For this review, take the finished solid that the model builds, in its own axes (mm). A direction names the side the tool comes from. Round coordinates to 2 decimals unless told otherwise and drop trailing zeros. Order: outer loops, then holes, each group sorted by start corner. A loop starts at its lowest first (then second) coordinate and runs counter-clockwise, first axis right, second up. Notation, with made-up numbers: (18.5, -23.5) -> (53.5, -23.5) arc R19 ccw to (53.5, 10.5) -> close; hole circle Ø9 at (44.25, 45.5). An arc over 180 degrees is marked (long way). Answer in a Markdown table with one row per item.
Autodesk Inventor part; units mm, degrees
ref_plane "YZ Plane" through (0, 0, 0) normal (1, 0, 0) x (0, 1, 0)
ref_plane "XZ Plane" through (0, 0, 0) normal (0, 1, 0) x (-1, 0, 0)
ref_plane "XY Plane" through (0, 0, 0) normal (0, 0, 1) x (1, 0, 0)
sketch "スケッチ1" plane through (0, 0, 0) normal (0, 1, 0) x (-1, 0, 0)
  circle A0 centre (0, 0) radius 2.75
  dimension "d0" = 5.5
extrude "押し出し1" add sketch "スケッチ1" along normal blind 3
sketch "スケッチ2" plane through (0, 0, 0) normal (0, -1, 0) x (1, 0, 0)
  circle A0 centre (0, 0) radius 1.5
  dimension "d3" = 3
extrude "押し出し2" add sketch "スケッチ2" along normal blind 8
fillet "フィレット1" radius 0.5 1 edges at (2.75, 3, 0)
fillet "フィレット1" radius 0.2 1 edges at (2.75, 0, 0)
sketch "スケッチ3" plane through (0, 3, 0) normal (0, 1, 0) x (1, 0, 0)
  line L0 (0, 1.4434) -> (-1.25, 0.7217)
  line L1 (-1.25, 0.7217) -> (-1.25, -0.7217)
  line L2 (-1.25, -0.7217) -> (0, -1.4434)
  line L3 (0, -1.4434) -> (1.25, -0.7217)
  line L4 (1.25, -0.7217) -> (1.25, 0.7217)
  line L5 (1.25, 0.7217) -> (0, 1.4434)
  line L6 (0, 1.4434) -> (0, -1.4434) construction
  circle A0 centre (0, 0) radius 1.4434 construction
  dimension "d12" = 2.5
extrude "押し出し3" cut sketch "スケッチ3" against normal blind 2
thread "ねじ1"
properties part number "M3-CapScrew"
Q1. Clearance check with flat-ended pins moving along their axes: pin 1 Ø1 at (y, z) = (-6, 1.5) entering from -X; pin 2 Ø0.7 at (y, z) = (1.5, -0.5) entering from -X; pin 3 Ø1.5 at (x, y) = (-2, 1) entering from +Z. State where each tip first meets the part, or that it passes through.
Answer key:
| item | result |
|---|---|
| pin 1 | stops at x = -1.12 |
| pin 2 | stops at x = -2.75 |
| pin 3 | stops at z = 2.45 |
Q2. To check wall thickness, follow probe 1 along X at (y, z) = (-3, -0.05); probe 2 along Y at (x, z) = (2.1, -0.4); probe 3 along Y at (x, z) = (0.15, 0.1). State the ranges of each line that lie inside material, in increasing order.
Answer key:
| item | result |
|---|---|
| probe 1 | x = -1.5 to 1.5 |
| probe 2 | y = 0 to 3 |
| probe 3 | y = -8 to 1 |
Q3. Take a section at A-A, the plane y = 1.5. Write out the cut boundary in (x, z), then the cut area to 3 significant figures.
Answer key:
| item | result |
|---|---|
| outline | circle Ø5.5 at (0, 0); hole (-1.25, -0.72) -> (0, -1.44) -> (1.25, -0.72) -> (1.25, 0.72) -> (0, 1.44) -> (-1.25, 0.72) -> close |
| area | 18.3 mm^2 |
Q4. Tool access review of faces 1 (the face through (0.63, 2.01, -1.08)), 2 (the face through (-2, 0, 0)), 3 (the face through (0, -8, 0)): name each direction out of +Z, -Z, +X, -X, +Y, -Y from which nothing blocks a thin tool from reaching the whole face with its end or side.
Answer key:
| item | result |
|---|---|
| face 1 | +Y |
| face 2 | -Y |
| face 3 | +Z, -Z, +X, -X, -Y |
Q5. Take a section at B-B, the plane z = 0. Write out the cut boundary in (x, y), then the cut area to 3 significant figures.
Answer key:
| item | result |
|---|---|
| outline | (-2.75, 0.2) arc R0.2 ccw to (-2.55, 0) -> (-1.5, 0) -> (-1.5, -8) -> (1.5, -8) -> (1.5, 0) -> (2.55, 0) arc R0.2 ccw to (2.75, 0.2) -> (2.75, 2.5) arc R0.5 ccw to (2.25, 3) -> (1.25, 3) -> (1.25, 1) -> (-1.25, 1) -> (-1.25, 3) -> (-2.25, 3) arc R0.5 ccw to (-2.75, 2.5) -> close |
| area | 35.4 mm^2 |
Q6. The part is to be moulded in two halves that separate along Z. For faces 4 (the face through (0.596, 1.334, 2.685)), 5 (the face through (-1.5, 3, 0)), 6 (the face through (0, 1, 0)), say which applies: +Z half, -Z half, draft (parallel to the pull), parting line (faces both ways), or undercut.
Answer key:
| item | result |
|---|---|
| face 4 | parting line |
| face 5 | draft |
| face 6 | undercut |
